Read the model definition and answer for the solid it produces. Units are mm, in the model's axes. Round coordinates to 2 decimals unless told otherwise and drop trailing zeros. Order: outer loops, then holes, each group sorted by start corner. A loop starts at its lowest first (then second) coordinate and runs counter-clockwise, first axis right, second up. Notation, with made-up numbers: (-2, 89) - (21, 89) arc R18 cw to (21, 108) - close; hole circle Ø1 at (15, 23.25). An arc over 180 degrees is marked (long way). Answer as a JSON object with one key per item and string values. Group by question number.
Q1. A cutting plane is placed at B-B on x = 64. Count the separate pieces of the cut face and the enclosed holes in it, and give its area (3 significant figures).
Q2. Consider line 1 (Y direction, x = -21.5, z = 1.3); line 2 (Y direction, x = 69, z = 4.7); line 3 (X direction, y = -40, z = 2.65). Determine where each line is inside the solid, lowest interval first.
Q3. Given pin 1 Ø1 at (x, z) = (-0.5, 0.5) entering from -Y, flat-ended and moving along its own axis, determine where the tip first touches the part or whether it passes through.
Q4. A cutting plane is placed at A-A on y = 9. Determine the outline of the cut face in (x, z), and give its area (3 significant figures).
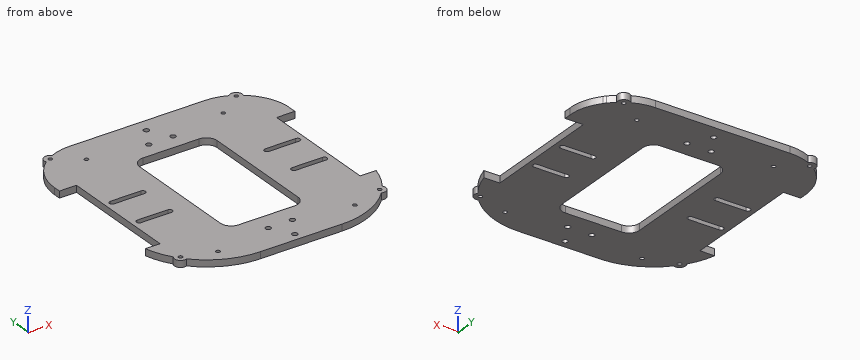
```python
from build123d import *

# Parameters (mm, degrees)
SKETCH1_R           = 2.01
SKETCH1_R_2         = 1.5
BOSS_EXTRUDE1_DEPTH = 5
SKETCH3_R           = 1.502108832
SKETCH3_R_2         = 1.5
CUT_EXTRUDE1_DEPTH  = 5
SKETCH6_R           = 127.388909146
CUT_EXTRUDE2_DEPTH  = 10
SKETCH7_R           = 1.5
CUT_EXTRUDE3_DEPTH  = 10
BOSS_EXTRUDE2_START = -5
SKETCH8_R           = 1.502108832
BOSS_EXTRUDE2_DEPTH = 5


with BuildPart() as part:
    # Sketch1 → Boss-Extrude1 (new body)
    with BuildSketch(Plane.XY):
        with BuildLine():
            Line((75.504557328, -44.459304845), (75.504557328, 45.540695166))
            Line((75.504557328, 45.540695166), (100.059689798, 45.540695166))
            add(Edge.make_bspline(
                [(100.059689798, 45.540695166), (100.041788228, 45.754261833), (99.850008352, 47.893495098), (98.96868948, 53.830439174), (96.130771714, 63.067301471), (90.671016468, 73.277711787), (83.341127235, 82.262457854), (74.36610438, 89.593910485), (64.164774078, 95.050161964), (54.928289046, 97.885319352), (47.287800195, 99.020154484), (43.400368962, 99.191158918), (41.462449937, 99.172959613)],
                knots=[0.055788601, 0.055788601, 0.055788601, 0.055788601, 0.062711167, 0.125182898, 0.250126359, 0.375069821, 0.500013282, 0.624956744, 0.749900205, 0.874843667, 0.937315398, 0.999787128, 0.999787128, 0.999787128, 0.999787128], degree=3))
            Line((41.462449937, 99.172959613), (-37.993292469, 99.172959613))
            add(Edge.make_bspline(
                [(-37.993292469, 99.172959613), (-41.828390734, 99.192174166), (-49.528051244, 98.435603453), (-60.581226949, 95.081607626), (-70.808859789, 89.670474861), (-79.808884098, 82.300210471), (-87.147846669, 73.275518481), (-92.643550681, 63.029136296), (-95.563376916, 53.601119233), (-96.412693125, 47.662538368), (-96.590112943, 45.540695166)],
                knots=[0.000114592, 0.000114592, 0.000114592, 0.000114592, 0.125060228, 0.250005865, 0.374951502, 0.499897139, 0.624842775, 0.749788412, 0.874734049, 0.943757473, 0.943757473, 0.943757473, 0.943757473], degree=3))
            Line((-96.590112943, 45.540695166), (-74.495442672, 45.540695166))
            Line((-74.495442672, 45.540695166), (-74.495442672, -44.459304845))
            Line((-74.495442672, -44.459304845), (-96.069812767, -44.459304845))
            Line((-96.069812767, -44.459304845), (-96.069812767, -58.94108417))
            add(Edge.make_bspline(
                [(-96.069812767, -58.94108417), (-96.103597655, -60.242783602), (-96.020757858, -62.86424422), (-95.284873318, -67.958362235), (-93.368947654, -74.058002404), (-89.696192927, -80.728467677), (-84.849845597, -86.58500717), (-79.007758993, -91.452906948), (-72.33795175, -95.146253023), (-66.222611962, -97.071224016), (-61.106429471, -97.805589863), (-58.468563645, -97.88419966), (-57.159547687, -97.847472391)],
                knots=[0.000901993, 0.000901993, 0.000901993, 0.000901993, 0.063285077, 0.12566816, 0.250434328, 0.375200496, 0.499966664, 0.624732831, 0.749498999, 0.874265167, 0.936648251, 0.999031335, 0.999031335, 0.999031335, 0.999031335], degree=3))
            Line((-57.159547687, -97.847472391), (62.058252081, -97.847472391))
            add(Edge.make_bspline(
                [(62.058252081, -97.847472391), (63.349284352, -97.87302538), (65.946474819, -97.778812963), (71.006373371, -97.039227825), (77.079986888, -95.147057025), (83.747716292, -91.525384678), (89.621452499, -86.731070085), (94.516764786, -80.923365419), (98.236814692, -74.255649702), (100.174956425, -68.105115813), (100.911947701, -62.938495931), (100.98924539, -60.262367482), (100.951464077, -58.935920146)],
                knots=[0.000693468, 0.000693468, 0.000693468, 0.000693468, 0.063089705, 0.125485942, 0.250278415, 0.375070889, 0.499863363, 0.624655837, 0.749448311, 0.874240785, 0.936637021, 0.999033258, 0.999033258, 0.999033258, 0.999033258], degree=3))
            Line((100.951464077, -58.935920146), (100.951464077, -44.459304845))
            Line((100.951464077, -44.459304845), (75.504557328, -44.459304845))
        make_face()
        with Locations((0.504557328, -81.923550041)):
            Circle(SKETCH1_R, mode=Mode.SUBTRACT)
        with Locations((-8.560442672, -66.22250947)):
            Circle(SKETCH1_R, mode=Mode.SUBTRACT)
        with Locations((9.569557328, -66.22250947)):
            Circle(SKETCH1_R, mode=Mode.SUBTRACT)
        with Locations(Location((9.569557328, 62.375409388, 0), (0, 0, 180))):
            Circle(SKETCH1_R, mode=Mode.SUBTRACT)
        with Locations(Location((-8.560442672, 62.375409388, 0), (0, 0, 180))):
            Circle(SKETCH1_R, mode=Mode.SUBTRACT)
        with Locations(Location((0.504557328, 78.076449959, 0), (0, 0, 180))):
            Circle(SKETCH1_R, mode=Mode.SUBTRACT)
        with Locations((51.787679438, 68.968213223)):
            Circle(SKETCH1_R_2, mode=Mode.SUBTRACT)
        with Locations(Location((-50.778564782, 68.968213223, 0), (0, 0, 180))):
            Circle(SKETCH1_R_2, mode=Mode.SUBTRACT)
        with Locations((-50.778564782, -72.815313305)):
            Circle(SKETCH1_R_2, mode=Mode.SUBTRACT)
        with Locations(Location((51.787679438, -72.815313305, 0), (0, 0, 180))):
            Circle(SKETCH1_R_2, mode=Mode.SUBTRACT)
        with BuildLine():
            Line((20.835255983, 50.556927645), (-21.225305639, 50.556927645))
            ThreePointArc((-21.225305639, 50.556927645), (-26.882159889, 48.213781894), (-29.225305639, 42.556927645))
            Line((-29.225305639, 42.556927645), (-29.225305639, -44.475522072))
            ThreePointArc((-29.225305639, -44.475522072), (-26.882159889, -50.132376322), (-21.225305639, -52.475522072))
            Line((-21.225305639, -52.475522072), (20.835255983, -52.475522072))
            ThreePointArc((20.835255983, -52.475522072), (26.492110233, -50.132376322), (28.835255983, -44.475522072))
            Line((28.835255983, -44.475522072), (28.835255983, 42.556927645))
            ThreePointArc((28.835255983, 42.556927645), (26.492110233, 48.213781894), (20.835255983, 50.556927645))
        make_face(mode=Mode.SUBTRACT)
        with BuildLine():
            Line((47.004557328, -15.95930484), (70.004557328, -15.95930484))
            ThreePointArc((70.004557328, -15.95930484), (72.004557328, -13.95930484), (70.004557328, -11.95930484))
            Line((70.004557328, -11.95930484), (47.004557328, -11.95930484))
            ThreePointArc((47.004557328, -11.95930484), (45.004557328, -13.95930484), (47.004557328, -15.95930484))
        make_face(mode=Mode.SUBTRACT)
        with BuildLine():
            Line((-45.995442672, -15.95930484), (-68.995442672, -15.95930484))
            ThreePointArc((-68.995442672, -15.95930484), (-70.995442672, -13.95930484), (-68.995442672, -11.95930484))
            Line((-68.995442672, -11.95930484), (-45.995442672, -11.95930484))
            ThreePointArc((-45.995442672, -11.95930484), (-43.995442672, -13.95930484), (-45.995442672, -15.95930484))
        make_face(mode=Mode.SUBTRACT)
        with BuildLine():
            Line((-45.995442672, 13.04069516), (-68.995442672, 13.04069516))
            ThreePointArc((-68.995442672, 13.04069516), (-70.995442672, 15.04069516), (-68.995442672, 17.04069516))
            Line((-68.995442672, 17.04069516), (-45.995442672, 17.04069516))
            ThreePointArc((-45.995442672, 17.04069516), (-43.995442672, 15.04069516), (-45.995442672, 13.04069516))
        make_face(mode=Mode.SUBTRACT)
        with BuildLine():
            Line((47.004557328, 13.04069516), (70.004557328, 13.04069516))
            ThreePointArc((70.004557328, 13.04069516), (72.004557328, 15.04069516), (70.004557328, 17.04069516))
            Line((70.004557328, 17.04069516), (47.004557328, 17.04069516))
            ThreePointArc((47.004557328, 17.04069516), (45.004557328, 15.04069516), (47.004557328, 13.04069516))
        make_face(mode=Mode.SUBTRACT)
    extrude(amount=BOSS_EXTRUDE1_DEPTH)

    # Sketch3 → Cut-Extrude1 (cut)
    with BuildSketch(Plane(origin=(-67.725712149, -284.067502755, 0), x_dir=(0, -1, 0), z_dir=(0, 0, -1))):
        with Locations(Location((-358.51234805, 8.035243007, 0), (0, 0, 90))):
            Circle(SKETCH3_R)
        with Locations(Location((-358.51234805, -146.964756993, 0), (0, 0, 90))):
            Circle(SKETCH3_R)
        with Locations(Location((-198.51234805, -146.964756993, 0), (0, 0, 90))):
            Circle(SKETCH3_R_2)
        with Locations(Location((-198.51234805, 8.035243007, 0), (0, 0, 90))):
            Circle(SKETCH3_R_2)
    extrude(amount=-CUT_EXTRUDE1_DEPTH, mode=Mode.SUBTRACT)

    # Sketch6 → Cut-Extrude2 (cut)
    with BuildSketch(Plane.XY.offset(5)):
        Circle(SKETCH6_R)
        with BuildLine():
            Line((-87.277351018, -30.425691892), (-87.277351018, 50.698917047))
            add(Edge.make_bspline(
                [(-87.277351018, 50.698917047), (-87.345293709, 62.092554876), (-81.91852953, 73.408536042), (-72.908806653, 80.366097079)],
                knots=[0, 0, 0, 0, 1, 1, 1, 1], degree=3))
            ThreePointArc((-72.908806653, 80.366097079), (-71.074769912, 85.869026234), (-65.340831928, 84.992741324))
            add(Edge.make_bspline(
                [(-65.340831928, 84.992741324), (-57.788055604, 88.493717217), (-49.542903418, 88.433129599)],
                knots=[0, 0, 0, 1, 1, 1], degree=2))
            Line((-49.542903418, 88.433129599), (51.441442769, 88.433129599))
            add(Edge.make_bspline(
                [(51.441442769, 88.433129599), (59.678483611, 88.437151289), (67.233362352, 84.98585913)],
                knots=[0, 0, 0, 1, 1, 1], degree=2))
            ThreePointArc((67.233362352, 84.98585913), (73.005560597, 85.849122489), (74.775204798, 80.287481041))
            add(Edge.make_bspline(
                [(74.775204798, 80.287481041), (83.589006393, 73.308525296), (89.668786675, 62.097481339), (89.175890368, 50.698917047)],
                knots=[0, 0, 0, 0, 1, 1, 1, 1], degree=3))
            Line((89.175890368, 50.698917047), (89.175890368, -30.425691892))
            add(Edge.make_bspline(
                [(89.175890368, -30.425691892), (89.178293605, -41.855069867), (85.762409509, -53.342513531), (79.252897634, -62.750515348)],
                knots=[0, 0, 0, 0, 1, 1, 1, 1], degree=3))
            ThreePointArc((79.252897634, -62.750515348), (79.128857618, -68.135420529), (73.929922922, -69.543847935))
            add(Edge.make_bspline(
                [(73.929922922, -69.543847935), (69.434477623, -74.486167285), (56.518819164, -84.02444032), (40.807367453, -88.132321569), (31.581207186, -88.020016316)],
                knots=[0, 0, 0, 0, 0.421407571, 1, 1, 1, 1], degree=3))
            Line((31.581207186, -88.020016316), (-29.682667836, -88.020016316))
            add(Edge.make_bspline(
                [(-29.682667836, -88.020016316), (-45.510843982, -88.093323652), (-61.333296445, -81.273069841), (-72.030941971, -69.543673037)],
                knots=[0, 0, 0, 0, 1, 1, 1, 1], degree=3))
            ThreePointArc((-72.030941971, -69.543673037), (-77.21426967, -68.155781128), (-77.38390991, -62.7925403))
            add(Edge.make_bspline(
                [(-77.38390991, -62.7925403), (-83.813349424, -53.321823673), (-87.323146284, -41.875751549), (-87.277351018, -30.425691892)],
                knots=[0, 0, 0, 0, 1, 1, 1, 1], degree=3))
        make_face(mode=Mode.SUBTRACT)
    extrude(amount=-CUT_EXTRUDE2_DEPTH, mode=Mode.SUBTRACT)

    # Sketch7 → Cut-Extrude3 (cut)
    with BuildSketch(Plane.XY.offset(5)):
        with Locations((75.586718904, -65.359946995)):
            Circle(SKETCH7_R)
        with Locations((-73.688179554, -65.359946995)):
            Circle(SKETCH7_R)
        with Locations((70.626130167, 82.029657757)):
            Circle(SKETCH7_R)
        with Locations((-68.727590817, 82.029657757)):
            Circle(SKETCH7_R)
    extrude(amount=-CUT_EXTRUDE3_DEPTH, mode=Mode.SUBTRACT)

    # Sketch8 → Boss-Extrude2 (add)
    with BuildSketch(Plane.XY.offset(5).offset(BOSS_EXTRUDE2_START)):
        with Locations((-75.760955156, 74.444845294)):
            Circle(SKETCH8_R)
        with BuildLine():
            ThreePointArc((79.425475108, 75.935340078), (78.101855611, 73.463452615), (80.740777557, 74.41123274))
            add(Edge.make_bspline(
                [(80.740777557, 74.41123274), (80.204403355, 75.278133212), (79.425475108, 75.935340078)],
                knots=[0, 0, 0, 1, 1, 1], degree=2))
        make_face()
    extrude(amount=BOSS_EXTRUDE2_DEPTH)


solid = part.part
```
Result set:
{
 "1": {"separate pieces": "3", "enclosed holes": "0", "area": "782 mm²"},
 "2": {"line 1": "y = -88.02 to -52.47, 50.55 to 88.43", "line 2": "y = -74.29 to -15.96, -11.96 to 13.04, 17.04 to 86.23", "line 3": "x = -74.5 to -29.23, 28.84 to 75.5"},
 "3": {"pin 1": "stops at y = -88.02"},
 "4": {"outline": "(-74.5, 0) - (-29.23, 0) - (-29.23, 5) - (-74.5, 5) - close; (28.84, 0) - (75.5, 0) - (75.5, 5) - (28.84, 5) - close", "area": "460 mm²"}
}
